from build123d import *

# Parameters (mm, degrees)
SKETCH_1_W          = 76.5
SKETCH_1_H          = 120
EXTRUDE_1_DEPTH     = 0.8
SKETCH_5_R          = 2.5
CUT_EXTRUDE_2_DEPTH = 143.31264877
SKETCH_7_R          = 4
SKETCH_7_R_2        = 2
EXTRUDE_2_DEPTH     = 5
SKETCH_8_W          = 22
SKETCH_8_H          = 32
CUT_EXTRUDE_4_DEPTH = 143.398209258
SKETCH_9_R          = 2
CUT_EXTRUDE_5_DEPTH = 143.398209258
SKETCH_10_W         = 69
SKETCH_10_H         = 112.5
SKETCH_10_W_2       = 67.4
SKETCH_10_H_2       = 110.9
EXTRUDE_4_DEPTH     = 5
SKETCH_11_W         = 0.8
SKETCH_11_H         = 30
CUT_EXTRUDE_6_DEPTH = 5
FILLET_1_R          = 2


with BuildPart() as part:
    # ｽｹｯﾁ1 → ﾎﾞｽ - 押し出し1 (new body)
    with BuildSketch(Plane.XY):
        with Locations((38.25, 60)):
            Rectangle(SKETCH_1_W, SKETCH_1_H)
    extrude(amount=EXTRUDE_1_DEPTH)

    # ｽｹｯﾁ5 → ｶｯﾄ - 押し出し2 (cut, through all)
    with BuildSketch(Plane.XY.offset(0.8)):
        with Locations((24, 65)):
            Circle(SKETCH_5_R)
        with Locations((24, 25)):
            Circle(SKETCH_5_R)
    extrude(amount=-CUT_EXTRUDE_2_DEPTH, mode=Mode.SUBTRACT)

    # ｽｹｯﾁ7 → ﾎﾞｽ - 押し出し2 (add)
    # profile 1 of 4: a face of its own
    with BuildSketch(Plane.XY.offset(0.8)):
        with Locations(Location((55, 80, 0), (0, 0, 180))):
            Circle(SKETCH_7_R)
        with Locations((55, 80)):
            Circle(SKETCH_7_R_2, mode=Mode.SUBTRACT)
    # profile 2 of 4: a face of its own
    with BuildSketch(Plane.XY.offset(0.8)):
        with Locations(Location((15, 80, 0), (0, 0, 180))):
            Circle(SKETCH_7_R)
        with Locations((15, 80)):
            Circle(SKETCH_7_R_2, mode=Mode.SUBTRACT)
    # profile 3 of 4: a face of its own
    with BuildSketch(Plane.XY.offset(0.8)):
        with Locations(Location((55, 10, 0), (0, 0, 180))):
            Circle(SKETCH_7_R)
        with Locations((55, 10)):
            Circle(SKETCH_7_R_2, mode=Mode.SUBTRACT)
    # profile 4 of 4: a face of its own
    with BuildSketch(Plane.XY.offset(0.8)):
        with Locations(Location((15, 10, 0), (0, 0, 180))):
            Circle(SKETCH_7_R)
        with Locations((15, 10)):
            Circle(SKETCH_7_R_2, mode=Mode.SUBTRACT)
    extrude(amount=EXTRUDE_2_DEPTH)

    # ｽｹｯﾁ8 → ｶｯﾄ - 押し出し4 (cut, through all)
    with BuildSketch(Plane.XY.offset(0.8)):
        with Locations((42, 45)):
            Rectangle(SKETCH_8_W, SKETCH_8_H)
    extrude(amount=-CUT_EXTRUDE_4_DEPTH, mode=Mode.SUBTRACT)

    # ｽｹｯﾁ9 → ｶｯﾄ - 押し出し5 (cut, through all)
    with BuildSketch(Plane.XY.offset(0.8)):
        with Locations((15, 80)):
            Circle(SKETCH_9_R)
        with Locations((55, 80)):
            Circle(SKETCH_9_R)
        with Locations((55, 10)):
            Circle(SKETCH_9_R)
        with Locations((15, 10)):
            Circle(SKETCH_9_R)
    extrude(amount=-CUT_EXTRUDE_5_DEPTH, mode=Mode.SUBTRACT)

    # ｽｹｯﾁ10 → ﾎﾞｽ - 押し出し4 (add)
    with BuildSketch(Plane.XY.offset(0.8)):
        with Locations((38.25, 60)):
            Rectangle(SKETCH_10_W, SKETCH_10_H)
        with Locations((38.25, 60)):
            Rectangle(SKETCH_10_W_2, SKETCH_10_H_2, mode=Mode.SUBTRACT)
    extrude(amount=EXTRUDE_4_DEPTH)

    # ｽｹｯﾁ11 → ｶｯﾄ - 押し出し6 (cut)
    with BuildSketch(Plane.XY.offset(5.8)):
        with Locations((72.35, 66.25)):
            Rectangle(SKETCH_11_W, SKETCH_11_H)
        Polygon((3.75, 116.25), (15.75, 116.25), (15.75, 115.45), (4.55, 115.45), (4.55, 104.25), (3.75, 104.25), align=None)
        Polygon((72.75, 104.25), (72.75, 116.25), (60.75, 116.25), (60.75, 115.45), (71.95, 115.45), (71.95, 104.25), align=None)
        Polygon((72.75, 3.75), (72.75, 15.75), (71.95, 15.75), (71.95, 4.55), (60.75, 4.55), (60.75, 3.75), align=None)
        Polygon((3.75, 3.75), (15.75, 3.75), (15.75, 4.55), (4.55, 4.55), (4.55, 15.75), (3.75, 15.75), align=None)
    extrude(amount=-CUT_EXTRUDE_6_DEPTH, mode=Mode.SUBTRACT)

    # ﾌｨﾚｯﾄ1
    # the kernel refuses this fillet: 2 mm, written as the material it adds along each edge
    with BuildSketch(Plane(origin=(60.75, 4.55, 0.8), x_dir=(0, 1, 0), z_dir=(-1, 0, 0)), Plane(origin=(15.75, 115.45, 0.8), x_dir=(0, -1, 0), z_dir=(1, 0, 0))) as fillet_1_piece_1:
        with BuildLine():
            CenterArc((FILLET_1_R, -FILLET_1_R), FILLET_1_R, 90, 90)
            Line((0, -FILLET_1_R), (0, 0))
            Line((0, 0), (FILLET_1_R, 0))
        make_face()
    extrude(amount=45)
    with BuildSketch(Plane(origin=(4.55, 15.75, 0.8), x_dir=(1, 0, 0), z_dir=(0, 1, 0))) as fillet_1_piece_2:
        with BuildLine():
            CenterArc((FILLET_1_R, -FILLET_1_R), FILLET_1_R, 90, 90)
            Line((0, -FILLET_1_R), (0, 0))
            Line((0, 0), (FILLET_1_R, 0))
        make_face()
    extrude(amount=88.5)
    with BuildSketch(Plane(origin=(71.95, 51.25, 0.8), x_dir=(-1, 0, 0), z_dir=(0, -1, 0))) as fillet_1_piece_3:
        with BuildLine():
            CenterArc((FILLET_1_R, -FILLET_1_R), FILLET_1_R, 90, 90)
            Line((0, -FILLET_1_R), (0, 0))
            Line((0, 0), (FILLET_1_R, 0))
        make_face()
    extrude(amount=35.5)
    with BuildSketch(Plane(origin=(71.95, 104.25, 0.8), x_dir=(-1, 0, 0), z_dir=(0, -1, 0))) as fillet_1_piece_4:
        with BuildLine():
            CenterArc((FILLET_1_R, -FILLET_1_R), FILLET_1_R, 90, 90)
            Line((0, -FILLET_1_R), (0, 0))
            Line((0, 0), (FILLET_1_R, 0))
        make_face()
    extrude(amount=23)


solid = part.part
Source: CAD feature listing. Evaluate the final solid. Frame: model axes, mm. A direction names the side the tool comes from. Round coordinates to 2 decimals unless told otherwise and drop trailing zeros. Loops run counter-clockwise (first coordinate to the right, second up) from the corner with the lowest first, then second, coordinate; pieces in that order, holes last. Notation, with made-up numbers: (15, -7.5) -> (30, -7.5) arc R34 ccw to (30, 31.5) -> close; hole circle Ø5 at (44.25, -30.5). An arc over 180 degrees is marked (long way). Answer as a JSON object with one key per item and string values. Group by question number.
Q1. Access query for faces 5 (the flat face through (4, 104.25, 3)), 6 (the flat face through (72.75, 93, 3)), 7 (the flat face through (38, 115.45, 4)). Directions: +Z, -Z, +X, -X, +Y, -Y. A direction counts if a zero-diameter tool reaches every point of the face in a straight line with its end or side. Return the directions, or none.
Q2. Section query A-A (y = 36). Output: boundary loops of the cut face in (x, z), plus the area to 3 significant figures.
Q3. Contact query for flat-ended pins moving along their axis: P1, Ø1.9, axis at y = 5.5, z = 4, coming from the -X side; P2, Ø3, axis at y = 115.5, z = 4, coming from the -X side; P3, Ø2, axis at x = 51.5, y = 17.5, coming from the +Z side. Output: stop coordinate, or through.
Q4. Section query B-B (x = 33.5). Output: boundary loops of the cut face in (y, z).
Q5. Section query C-C (y = 80). Output: boundary loops of the cut face in (x, z), plus the area to 3 significant figures.
Q6. Mould query, pull axis Y, two halves, no side actions, for faces 1 (the cylindrical face through (21.5, 65.1, 0.4)), 2 (the flat face through (15.75, 4, 3)), 3 (the cylindrical face through (15.867, 83.905, 3.265)), 4 (the flat face through (72.3, 104.25, 3.3)). Classes: pulls with the +Y half, pulls with the -Y half, needs draft (parallel to the pull), parting line crosses it, or undercut.
Q7. Section query D-D (y = 65). Output: boundary loops of the cut face in (x, z).
Q8. Ray query, line 1 (Y direction, x = 15, z = 0.5); line 2 (Y direction, x = 55, z = 3.3); line 3 (Y direction, x = 15, z = 2.1). Return the intervals inside material, ascending. Write a range as from..to.
Completed:
{
 "1": {"face 5": "+Z, +X, -X, +Y", "face 6": "+Z, +X, +Y, -Y", "face 7": "+Z, +X, -X"},
 "2": {"outline": "(0, 0) -> (31, 0) -> (31, 0.8) -> (6.55, 0.8) arc R2 cw to (4.55, 2.8) -> (4.55, 5.8) -> (3.75, 5.8) -> (3.75, 0.8) -> (0, 0.8) -> close; (53, 0) -> (76.5, 0) -> (76.5, 0.8) -> (72.75, 0.8) -> (72.75, 5.8) -> (71.95, 5.8) -> (71.95, 2.8) arc R2 cw to (69.95, 0.8) -> (53, 0.8) -> close", "area": "53.3 mm²"},
 "3": {"P1": "x = 13.16", "P2": "x = 15.75", "P3": "z = 0.8"},
 "4": {"outline": "(0, 0) -> (29, 0) -> (29, 0.8) -> (6.55, 0.8) arc R2 cw to (4.55, 2.8) -> (4.55, 5.8) -> (3.75, 5.8) -> (3.75, 0.8) -> (0, 0.8) -> close; (61, 0) -> (120, 0) -> (120, 0.8) -> (116.25, 0.8) -> (116.25, 5.8) -> (115.45, 5.8) -> (115.45, 2.8) arc R2 cw to (113.45, 0.8) -> (61, 0.8) -> close"},
 "5": {"outline": "(0, 0) -> (13, 0) -> (13, 5.8) -> (11, 5.8) -> (11, 0.8) -> (6.55, 0.8) arc R2 cw to (4.55, 2.8) -> (4.55, 5.8) -> (3.75, 5.8) -> (3.75, 0.8) -> (0, 0.8) -> close; (17, 0) -> (53, 0) -> (53, 5.8) -> (51, 5.8) -> (51, 0.8) -> (19, 0.8) -> (19, 5.8) -> (17, 5.8) -> close; (57, 0) -> (76.5, 0) -> (76.5, 0.8) -> (59, 0.8) -> (59, 5.8) -> (57, 5.8) -> close", "area": "99.7 mm²"},
 "6": {"face 1": "undercut", "face 2": "needs draft", "face 3": "undercut", "face 4": "pulls with the +Y half"},
 "7": {"outline": "(0, 0) -> (21.5, 0) -> (21.5, 0.8) -> (6.55, 0.8) arc R2 cw to (4.55, 2.8) -> (4.55, 5.8) -> (3.75, 5.8) -> (3.75, 0.8) -> (0, 0.8) -> close; (26.5, 0) -> (76.5, 0) -> (76.5, 0.8) -> (26.5, 0.8) -> close"},
 "8": {"line 1": "0..8, 12..78, 82..120", "line 2": "3.75..4.55, 6..8, 12..14, 76..78, 82..84, 115.45..116.25", "line 3": "6..8, 12..14, 76..78, 82..84"}
}
